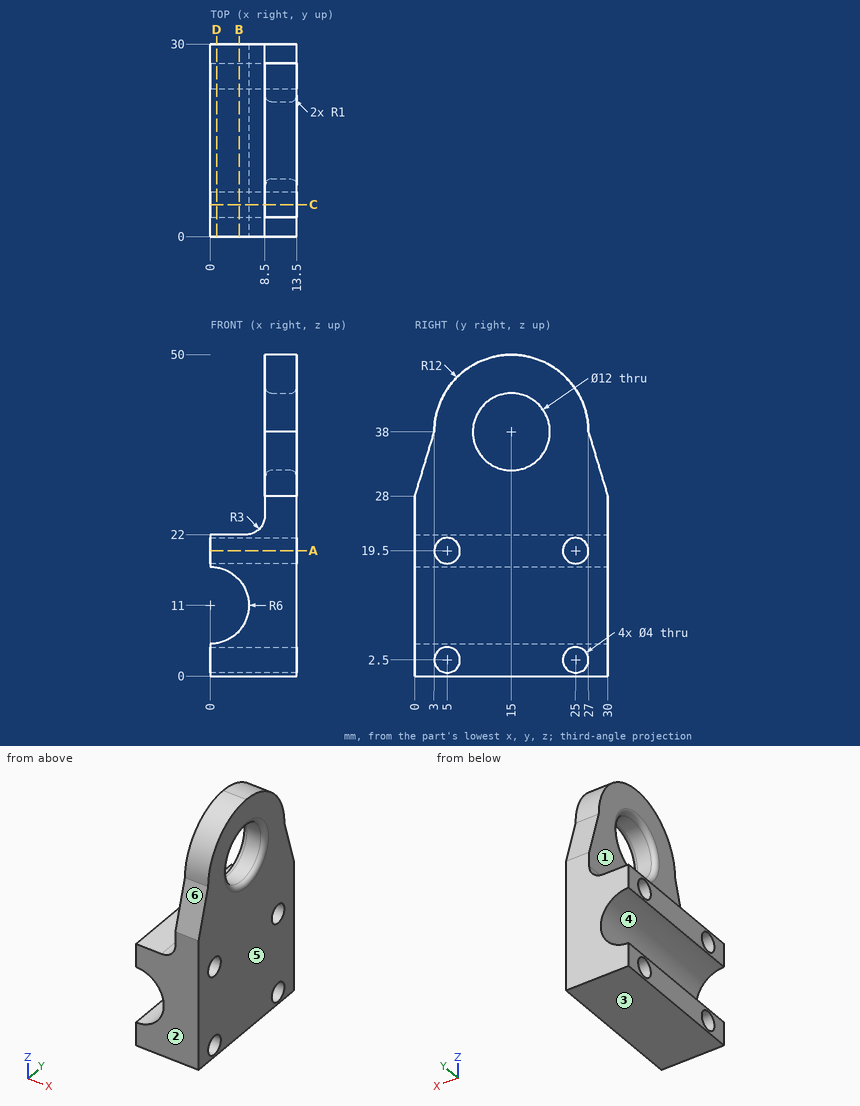
Print and shaded views of the part. All mm, measured from the part's lowest x, y and z. A direction names the side the tool comes from. Round coordinates to 2 decimals unless told otherwise and drop trailing zeros. Write each loop counter-clockwise with the first axis right and the second up, starting at its lowest first coordinate (ties: lowest second). Pieces come first, ordered by that corner, then holes. Notation, with made-up numbers: (23, 19.25) - (39, 19.25) arc R9 ccw to (39, 27.25) - close; hole circle Ø2 at (46, 79). An arc over 180 degrees is marked (long way). One line per question, with ' | ' between items.
1. Drill centre lines: line 1 along Y through (x, z) = (5.5, 2.5); line 2 along Y through (x, z) = (12.5, 4); line 3 along X through (y, z) = (21.25, 25). Where is each one in solid material? Low to high. Write a range as from..to.
Results are:
line 1: 0..3, 7..23, 27..30 | line 2: 0..3.68, 6.32..23.68, 26.32..30 | line 3: 8.5..13.5
2. Tool access for the marked faces 1 and 2: list every direction of +Z, -Z, +X, -X, +Y, -Y with a clear straight run to the whole face (end or side of a thin tool).
Results are:
face 1: +Z, -X, +Y, -Y | face 2: +Z, -Z, +X, -X, -Y
3. Mould opens along Z. For the marked faces 3, 4, 5 and 6 say: released by +Z, released by -Z, zero draft, split by the parting line, or undercut.
Results are:
face 3: released by -Z | face 4: undercut | face 5: zero draft | face 6: released by +Z
4. Band-saw the part on A-A, the plane z = 19.5. Write the cut outline in (x, y), and give its area (3 significant figures).
Results are:
outline: (0, 0) - (13.5, 0) - (13.5, 3) - (0, 3) - close; (0, 7) - (13.5, 7) - (13.5, 23) - (0, 23) - close; (0, 27) - (13.5, 27) - (13.5, 30) - (0, 30) - close | area: 297 mm^2
5. Band-saw the part on D-D, the plane x = 1. Write the cut outline in (y, z), and give its area (3 significant figures).
Results are:
outline: (0, 0) - (30, 0) - (30, 5.08) - (0, 5.08) - close; (0, 16.92) - (30, 16.92) - (30, 22) - (0, 22) - close; hole circle Ø4 at (5, 2.5); hole circle Ø4 at (5, 19.5); hole circle Ø4 at (25, 2.5); hole circle Ø4 at (25, 19.5) | area: 255 mm^2
6. Band-saw the part on C-C, the plane y = 5. Write the cut outline in (x, z), and give its area (3 significant figures).
Results are:
outline: (0, 0) - (13.5, 0) - (13.5, 0.5) - (0, 0.5) - close; (0, 4.5) - (13.5, 4.5) - (13.5, 17.5) - (0, 17.5) - (0, 17) arc R6 cw to (0, 5) - close; (0, 21.5) - (13.5, 21.5) - (13.5, 44.63) - (8.5, 44.63) - (8.5, 25) arc R3 cw to (5.5, 22) - (0, 22) - close | area: 248 mm^2
7. Band-saw the part on B-B, the plane x = 4.5. Write the cut outline in (y, z).
Results are:
outline: (0, 0) - (30, 0) - (30, 7.03) - (0, 7.03) - close; (0, 14.97) - (30, 14.97) - (30, 22) - (0, 22) - close; hole circle Ø4 at (5, 2.5); hole circle Ø4 at (5, 19.5); hole circle Ø4 at (25, 2.5); hole circle Ø4 at (25, 19.5)
8. Drop flat-ended pins along their axis: pin 1 Ø3 at (x, y) = (2, 18) entering from +Z; pin 2 Ø4 at (y, z) = (4, 29.5) entering from -X; pin 3 Ø7.5 at (y, z) = (15, 40.5) entering from -X. Give the stop position or say it passes through.
Results are:
pin 1: z = 22 | pin 2: x = 8.5 | pin 3: x = 8.84
